from build123d import *

# Parameters (mm, degrees)
BOSS_EXTRUDE1_DEPTH                                 = 8
BOSS_EXTRUDE2_DEPTH                                 = 3
CUT_EXTRUDE1_START                                  = -4
SKETCH13_W                                          = 15.2
SKETCH13_H                                          = 15.2
CUT_EXTRUDE1_DEPTH                                  = 4
FILLET1_R                                           = 2
SKETCH14_R                                          = 5
CUT_EXTRUDE4_DEPTH                                  = 126.924580603
M2_TAPPED_HOLE1_D                                   = 1.6
CUT_EXTRUDE5_DEPTH                                  = 126.924580603
M2_5_TAPPED_HOLE1_D                                 = 2.05
M2_5_TAPPED_HOLE1_DEPTH                             = 7.25
M2_5_TAPPED_HOLE1_TIP                               = 0.615882135
CSK_FOR_M5_COUNTERSUNK_FLAT_HEAD_SCREW1_D           = 5.1
CSK_FOR_M5_COUNTERSUNK_FLAT_HEAD_SCREW1_CSINK_D     = 10.4
CSK_FOR_M5_COUNTERSUNK_FLAT_HEAD_SCREW1_CSINK_ANGLE = 90


with BuildPart() as part:
    # Sketch3 → Boss-Extrude1 (new body)
    with BuildSketch(Plane(origin=(0, 0, 0), x_dir=(-1, 0, 0), z_dir=(0, 0, -1))):
        with BuildLine():
            Line((-70, 0), (70, 0))
            Line((70, 0), (70, 99))
            ThreePointArc((70, 99), (69.414213562, 100.414213562), (68, 101))
            Line((68, 101), (-68, 101))
            ThreePointArc((-68, 101), (-69.414213562, 100.414213562), (-70, 99))
            Line((-70, 99), (-70, 0))
        make_face()
    extrude(amount=BOSS_EXTRUDE1_DEPTH)

    # Sketch4 → Boss-Extrude2 (add)
    with BuildSketch(Plane(origin=(0, 0, -8), x_dir=(-1, 0, 0), z_dir=(0, 0, -1))):
        with BuildLine():
            Line((-72, 0), (72, 0))
            Line((72, 0), (72, 99))
            ThreePointArc((72, 99), (70.828427125, 101.828427125), (68, 103))
            Line((68, 103), (-68, 103))
            ThreePointArc((-68, 103), (-70.828427125, 101.828427125), (-72, 99))
            Line((-72, 99), (-72, 0))
        make_face()
    extrude(amount=-BOSS_EXTRUDE2_DEPTH)

    # Sketch5 → CSK for M4 Countersunk Flat Head Screw1 (revolve, cut)
    with BuildSketch(Plane(origin=(40, 10, -8), x_dir=(0, 1, 0), z_dir=(1, 0, 0))):
        Polygon((0, 0), (0, 8), (2.25, 8), (2.25, 3.45), (4.7, 1), (4.7, 0), align=None)
    csk_for_m4_countersunk_flat_head_screw1 = revolve(axis=Axis((40, 10, -14.35), (0, 0, 1)), mode=Mode.SUBTRACT)

    # Mirror1: CSK for M4 Countersunk Flat Head Screw1 across plane
    add(csk_for_m4_countersunk_flat_head_screw1.mirror(Plane(origin=(0, 0, 0), x_dir=(0, 0, 1), z_dir=(1, 0, 0))), mode=Mode.SUBTRACT)

    # Sketch13 → Cut-Extrude1 (cut)
    with BuildSketch(Plane(origin=(0, 0, -8), x_dir=(-1, 0, 0), z_dir=(0, 0, -1)).offset(CUT_EXTRUDE1_START)):
        with Locations((-0.5, 60)):
            Rectangle(SKETCH13_W, SKETCH13_H)
    extrude(amount=CUT_EXTRUDE1_DEPTH, mode=Mode.SUBTRACT)

    # Fillet1
    fillet1_edges = [part.edges().sort_by_distance(p)[0] for p in [
        (8.1, 67.6, -6),
        (8.1, 52.4, -6),
        (-7.1, 52.4, -6),
        (-7.1, 67.6, -6),
    ]]
    fillet(fillet1_edges, radius=FILLET1_R)

    # Sketch14 → Cut-Extrude4 (cut, through all)
    with BuildSketch(Plane(origin=(0, 0, -8), x_dir=(-1, 0, 0), z_dir=(0, 0, -1))):
        with Locations((-0.5, 60)):
            Circle(SKETCH14_R)
    extrude(amount=-CUT_EXTRUDE4_DEPTH, mode=Mode.SUBTRACT)

    # M2 Tapped Hole1 (through all)
    with Locations(Plane(origin=(0, 0, -4), x_dir=(-1, 0, 0), z_dir=(0, 0, -1))):
        with Locations((4.25, 64.75), (-5.25, 55.25)):
            Hole(M2_TAPPED_HOLE1_D / 2)

    # DB conn slot → Cut-Extrude5 (cut, through all)
    with BuildSketch(Plane(origin=(0, 0, -8), x_dir=(-1, 0, 0), z_dir=(0, 0, -1))):
        with BuildLine():
            Line((-56.5, 29.25), (-17.5, 29.25))
            ThreePointArc((-17.5, 29.25), (-16.439339828, 29.689339828), (-16, 30.75))
            Line((-16, 30.75), (-16, 39.25))
            ThreePointArc((-16, 39.25), (-16.439339828, 40.310660172), (-17.5, 40.75))
            Line((-17.5, 40.75), (-56.5, 40.75))
            ThreePointArc((-56.5, 40.75), (-57.560660172, 40.310660172), (-58, 39.25))
            Line((-58, 39.25), (-58, 30.75))
            ThreePointArc((-58, 30.75), (-57.560660172, 29.689339828), (-56.5, 29.25))
        make_face()
    extrude(amount=-CUT_EXTRUDE5_DEPTH, mode=Mode.SUBTRACT)

    # M2.5 Tapped Hole1
    with Locations(Plane(origin=(0, 0, -8), x_dir=(-1, 0, 0), z_dir=(0, 0, -1))):
        with Locations((-60.75, 35), (-13.25, 35)):
            Hole(M2_5_TAPPED_HOLE1_D / 2, depth=M2_5_TAPPED_HOLE1_DEPTH)
            with Locations((0, 0, -(M2_5_TAPPED_HOLE1_DEPTH + M2_5_TAPPED_HOLE1_TIP / 2))):  # 118° drill point
                Cone(0, M2_5_TAPPED_HOLE1_D / 2, M2_5_TAPPED_HOLE1_TIP, mode=Mode.SUBTRACT)

    # CSK for M5 Countersunk Flat Head Screw1 (through all)
    with Locations(Plane(origin=(0, 0, -8), x_dir=(-1, 0, 0), z_dir=(0, 0, -1))):
        with Locations((-37, 55)):
            CounterSinkHole(CSK_FOR_M5_COUNTERSUNK_FLAT_HEAD_SCREW1_D / 2, CSK_FOR_M5_COUNTERSUNK_FLAT_HEAD_SCREW1_CSINK_D / 2, counter_sink_angle=CSK_FOR_M5_COUNTERSUNK_FLAT_HEAD_SCREW1_CSINK_ANGLE)


solid = part.part
Here's how the part is built. I have some questions about the finished solid (model axes, mm). A direction names the side the tool comes from. Give positions to 0.01 mm unless a question says otherwise; leave off trailing zeros. Order: outer loops, then holes, each group sorted by start corner. A loop starts at its lowest first (then second) coordinate and runs counter-clockwise, first axis right, second up. Notation, with made-up numbers: (-20.5, -34) -> (32.5, -34) arc R6 ccw to (32.5, -28) -> close; hole circle Ø2 at (-2, -39.5). An arc over 180 degrees is marked (long way). Use a Markdown table: item, result. Add a question column.
Item 1: For faces 5 (the face through (58, 35, -4)), 6 (the face through (1, 67.6, -6)), 7 (the face through (-70.859, 101.797, -6.521)), which set-ups out of +Z, -Z, +X, -X, +Y, -Y let a thin tool reach every point of the face, with its end or its side?
Item 2: I need wall thicknesses on line 1 (Y direction, x = 37, z = -3.5); line 2 (X direction, y = 10, z = -7.7); line 3 (X direction, y = 10, z = -2.15). Which ranges of each line are inside material? Lowest first, please.
Item 3: If we mould it in two halves opening along X, with no side actions, what happens to faces 1 (the face through (1, 51, 0)), 2 (the face through (70, 50, -2)), 3 (the face through (34.3, 55.1, -5.5)), 4 (the face through (-70, 49, -2))? For each: pulls with the +X half, pulls with the -X half, needs draft (parallel to the pull), parting line crosses it, or undercut.
Item 4: Imagine slicing it at A-A on x = 22.5. Please give me the cut outline in (y, z), plus the area to 3 significant figures.
Item 5: Imagine slicing it at B-B on y = 77. Please give me the cut outline in (x, z).
Item 6: Will these pins go through, and if not, where does the flat tip stop? pin 1 (1.5 mm diameter, centred on y = 22, z = -2, fed in from +X); pin 2 (1.8 mm diameter, centred on x = -4.25, y = 64.75, fed in from -Z); pin 3 (8.5 mm diameter, centred on x = 40, y = 10, fed in from -Z).
Data:
| question | item | result |
|---|---|---|
| 1 | face 5 | +Z, -Z |
| 1 | face 6 | -Z |
| 1 | face 7 | +Z, -Z, -X, +Y |
| 2 | line 1 | y = 0 to 29.25, 40.75 to 52.45, 57.55 to 101 |
| 2 | line 2 | x = -72 to -44.7, -35.3 to 35.3, 44.7 to 72 |
| 2 | line 3 | x = -70 to -42.25, -37.75 to 37.75, 42.25 to 70 |
| 3 | face 1 | needs draft |
| 3 | face 2 | pulls with the +X half |
| 3 | face 3 | undercut |
| 3 | face 4 | pulls with the -X half |
| 4 | outline | (0, -8) -> (29.25, -8) -> (29.25, 0) -> (0, 0) -> close; (40.75, -8) -> (103, -8) -> (103, -5) -> (101, -5) -> (101, 0) -> (40.75, 0) -> close |
| 4 | area | 722 mm² |
| 5 | outline | (-72, -8) -> (72, -8) -> (72, -5) -> (70, -5) -> (70, 0) -> (-70, 0) -> (-70, -5) -> (-72, -5) -> close |
| 6 | pin 1 | stops at x = 70 |
| 6 | pin 2 | stops at z = -4 |
| 6 | pin 3 | stops at z = -6.55 |
